from build123d import *

# Parameters (mm, degrees)
BOSS_EXTRUDE1_DEPTH = 20
CUT_EXTRUDE1_DEPTH  = 15
FILLET1_R           = 2
SKETCH3_R           = 1.5
CUT_EXTRUDE2_DEPTH  = 31.083311404
SKETCH4_R           = 1.5
CUT_EXTRUDE3_DEPTH  = 31.083311404


with BuildPart() as part:
    # Sketch1 → Boss-Extrude1 (new body)
    with BuildSketch(Plane(origin=(0, 0, 0), x_dir=(0, 0, -1), z_dir=(1, 0, 0))):
        Polygon((0, -12.5), (-3.175, -12.5), (-6.175, -12.5), (-6.175, 6.175), (12.5, 6.175), (12.5, 3.175), (12.5, 0), (12.5, -3), (3, -12.5), align=None)
    extrude(amount=BOSS_EXTRUDE1_DEPTH)

    # Sketch2 → Cut-Extrude1 (cut)
    with BuildSketch(Plane(origin=(20, 0, 0), x_dir=(0, 0, -1), z_dir=(1, 0, 0))):
        Polygon((-3.175, -12.5), (0, -12.5), (0, 0), (12.5, 0), (12.5, 3.175), (-3.175, 3.175), align=None)
    extrude(amount=-CUT_EXTRUDE1_DEPTH, mode=Mode.SUBTRACT)

    # Fillet1
    fillet1_edges = [part.edges().sort_by_distance(p)[0] for p in [
        (20, -4.6625, 3.175),
        (20, -6.25, 0),
        (20, 0, -6.25),
        (20, 3.175, -4.6625),
    ]]
    fillet(fillet1_edges, radius=FILLET1_R)

    # Sketch3 → Cut-Extrude2 (cut, through all)
    with BuildSketch(Plane(origin=(0, 6.175, 0), x_dir=(1, 0, 0), z_dir=(0, 1, 0))):
        with Locations(Location((12.5, 6, 0), (0, 0, 90))):
            Circle(SKETCH3_R)
    extrude(amount=-CUT_EXTRUDE2_DEPTH, mode=Mode.SUBTRACT)

    # Sketch4 → Cut-Extrude3 (cut, through all)
    with BuildSketch(Plane.XY.offset(6.175)):
        with Locations((12.5, -6)):
            Circle(SKETCH4_R)
    extrude(amount=-CUT_EXTRUDE3_DEPTH, mode=Mode.SUBTRACT)


solid = part.part
Work out the finished part from the listing and answer in its coordinate system (mm). A direction names the side the tool comes from. Coordinates: 2 decimals unless noted, no trailing zeros. Write each loop counter-clockwise with the first axis right and the second up, starting at its lowest first coordinate (ties: lowest second). Pieces come first, ordered by that corner, then holes. Notation, with made-up numbers: (32.25, 22) - (85.25, 22) arc R12 ccw to (85.25, 31) - close; hole circle Ø4 at (22, 26.5). An arc over 180 degrees is marked (long way). One line per question, with ' | ' between items.
1) Flat-ended cylindrical pins translate along their axes: P1, Ø3.5, axis at x = 12.5, y = -6, coming from the -Z side; P2, Ø3.5, axis at x = 12.5, z = -6, coming from the -Y side; P3, Ø4, axis at x = 9, y = -8.5, coming from the -Z side. Find the tip coordinate at first contact, or state that the pin passes through.
Checks:
P1: z = -11.25 | P2: y = -11.25 | P3: z = -9
2) Find section B-B, the plane x = 10.5. Determine the outline of the cut face in (y, z) (3 decimals), and give its area (3 significant figures).
Checks:
outline: (-12.5, -3) - (-3, -12.5) - (0, -12.5) - (0, 0) - (-12.5, 0) - close; (-12.5, 3.175) - (3.175, 3.175) - (3.175, -12.5) - (6.175, -12.5) - (6.175, 6.175) - (-12.5, 6.175) - close | area: 214 mm2
3) Find section D-D, the plane y = 2.5. Determine the outline of the cut face in (x, z) (3 decimals), and give its area (3 significant figures).
Checks:
outline: (0, -12.5) - (5, -12.5) - (5, 3.175) - (18, 3.175) arc R2 ccw to (20, 5.175) - (20, 6.175) - (0, 6.175) - close | area: 138 mm2
4) Find section A-A, the plane x = 12.5. Give the number of separate pieces and of enclosed holes in the cut face, and give its area (3 significant figures).
Checks:
separate pieces: 7 | enclosed holes: 0 | area: 148 mm2
5) Find section C-C, the plane z = -2.5. Determine the outline of the cut face in (x, y) (3 decimals), and give its area (3 significant figures).
Checks:
outline: (0, -12.5) - (20, -12.5) - (20, -2) arc R2 ccw to (18, 0) - (5, 0) - (5, 3.175) - (18, 3.175) arc R2 ccw to (20, 5.175) - (20, 6.175) - (0, 6.175) - close; hole circle Ø3 at (12.5, -6) | area: 317 mm2
6) For faces 5 (the face through (0, -3, -3)), 6 (the face through (19.399, -3.786, 3.745)), 7 (the face through (19.43, 3.776, -3.539)), determine the directions among +Z, -Z, +X, -X, +Y, -Y from which every point of the face is accessible in a straight line to the end or side of a thin tool.
Checks:
face 5: +Z, -Z, -X, +Y, -Y | face 6: +X, -Y | face 7: -Z, +X
7) Consider probe 1 along Y at (x, z) = (12.5, 5.6) (3 decimals); probe 2 along X at (y, z) = (-6, -7.25). Determine where each line is inside the solid, lowest interval first. Write a range as [from, to].
Checks:
probe 1: [-12.5, -7.5], [-4.5, 6.175] | probe 2: [0, 11], [14, 20]
8) The mould has two halves that part along Y. Classify faces 1 (the face through (10, 4, -12.5)), 2 (the face through (12.305, -4.513, -8.483)), 3 (the face through (10, 3.175, -5)), 4 (the face through (9.9, -7.7, -7.8)): +Y half, -Y half, draft (parallel to the pull), parting line (faces both ways), or undercut.
Checks:
face 1: draft | face 2: undercut | face 3: undercut | face 4: -Y half
